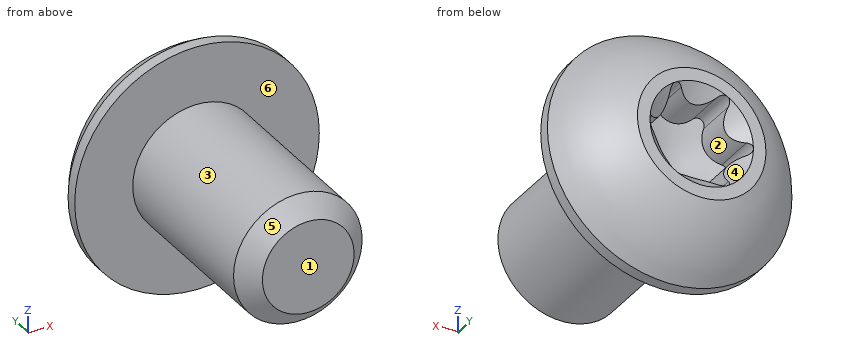
Autodesk Inventor part; units mm, degrees
ref_plane "YZ Plane" through (0, 0, 0) normal (1, 0, 0) x (0, 1, 0)
ref_plane "XZ Plane" through (0, 0, 0) normal (0, 1, 0) x (-1, 0, 0)
ref_plane "XY Plane" through (0, 0, 0) normal (0, 0, 1) x (1, 0, 0)
sketch "Sketch1" plane through (0, 0, 0) normal (0, 1, 0) x (-1, 0, 0)
  circle A0 centre (0, 0) radius 2.0828
  dimension "d4" = 4.1656
extrude "Body" add sketch "Sketch1" along normal blind 6.35
sketch "Sketch2" plane through (0, 0, 0) normal (1, 0, 0) x (0, 1, 0)
  line L0 (6.35, -2.0828) -> (6.35, 2.0828)
  line L1 (6.35, 0) -> (6.35, -3.9624)
  line L2 (6.35, -3.9624) -> (6.731, -3.9624)
  arc A0 (6.731, -3.9624) -> (8.5598, -2.0828) centre (4.5388, 0) ccw
  line L3 (8.5598, -2.0828) -> (8.5598, -1.6764)
  line L4 (8.5598, -1.6764) -> (7.0635, -1.6764)
  line L5 (7.0635, -1.6764) -> (6.4516, 0)
  line L6 (6.4516, 0) -> (6.35, 0)
  point P0 (0, 0)
  dimension "d5" = 3.9624
  dimension "d6" = 0.381
  dimension "d13" = 0.1016
  dimension "d14" = 2.0828
  dimension "d15" = 2.2098
  dimension "d16" = 0
  dimension "d17" = 1.6764
  dimension "d57" = 20.053
revolve "Head" add sketch "Sketch2" angle 360 about axis through (0, 6.4516, 0) along (0, -1, 0)
sketch "Sketch3" plane through (0, 8.5598, 0) normal (0, 1, 0) x (1, 0, 0)
  circle A0 centre (0, 0) radius 1.6764
  line L0 (0.7302, -1.2648) -> (-0.7303, -1.2648) construction
  line L1 (-0.7303, -1.2648) -> (-1.4605, 0) construction
  line L2 (-1.4605, 0) -> (-0.7303, 1.2648) construction
  line L3 (-0.7303, 1.2648) -> (0.7302, 1.2648) construction
  line L4 (0.7302, 1.2648) -> (1.4605, 0) construction
  line L5 (1.4605, 0) -> (0.7302, -1.2648) construction
  circle A1 centre (-0.7303, -1.2648) radius 0.2159
  circle A2 centre (-1.4605, 0) radius 0.2159
  circle A3 centre (-0.7303, 1.2648) radius 0.2159
  circle A4 centre (0.7302, 1.2648) radius 0.2159
  circle A5 centre (1.4605, 0) radius 0.2159
  circle A6 centre (0.7302, -1.2648) radius 0.2159
  circle A7 centre (0, -2.0701) radius 0.8712
  circle A8 centre (0, 2.0701) radius 0.8712
  circle A9 centre (1.7928, -1.0351) radius 0.8712
  circle A10 centre (-1.7928, 1.035) radius 0.8712
  circle A11 centre (1.7928, 1.035) radius 0.8712
  circle A12 centre (-1.7928, -1.0351) radius 0.8712
  circle A13 centre (0, 0) radius 1.8188
  point P0 (0, 0)
  point P1 (0, 0)
  point P2 (0.9413, 1.2192)
  point P3 (1.5265, 0.2056)
  point P4 (1.5265, -0.2056)
  point P5 (0.9413, -1.2192)
  point P6 (0.5852, -1.4248)
  point P7 (-0.5852, -1.4248)
  point P8 (-0.9413, -1.2192)
  point P9 (-1.5265, -0.2056)
  point P10 (-1.5265, 0.2056)
  point P11 (-0.9413, 1.2192)
  point P12 (-0.5852, 1.4248)
  point P13 (0.5852, 1.4248)
  dimension "d58" = 2.921
  dimension "d59" = 4.1402
  dimension "d62" = 120
extrude "Hex" add sketch "Sketch3" against normal blind 1.778 contours A5 A11 A0 | A0 A11 A13 A9 | A0 A9 A5 | A11 A0 | A0 A11 A13 | A9 A13 A0 | A0 A9 | A11 A4 A0 | A0 A8 A13 A11 | A9 A13 A7 A0 | A0 A6 A9 | A4 A8 A0 | A0 A7 A6 | A8 A0 | A7 A0 | A0 A8 A13 | A7 A13 A0 | A3 A0 A8 | A7 A0 A1 | A0 A10 A13 A8 | A7 A13 A12 A0 | A3 A10 A0 | A0 A12 A1 | A10 A0 A13 | A13 A12 A0 | A10 A0 | A0 A12 | A10 A0 A12 A13 | A10 A2 A0 | A0 A2 A12
sketch "Sketch4" plane through (0, 0, 0) normal (0, 0, 1) x (1, 0, 0)
  line L0 (-0.7364, 7.6198) -> (-1.6764, 8.5598)
  line L1 (0, 8.5598) -> (-0.7364, 7.6198)
  line L2 (0, -3.617) -> (0, 21.7018)
  line L3 (-1.5265, 8.5598) -> (-1.5265, 7.0138)
  line L4 (-1.5265, 8.5598) -> (-1.5265, 8.5598)
  line L5 (-1.5265, 8.5598) -> (-1.5265, 7.0138)
  line L6 (-1.6764, 8.5598) -> (-1.5265, 8.5598)
  line L7 (-1.6764, 8.5598) -> (0, 8.5598)
  point P0 (0, 0)
  point P1 (-1.6764, 7.0635)
  dimension "d29" = 1.6764
revolve "Head Chamfer" cut sketch "Sketch4" angle 360 about axis through (0, -10, 0) along (0, 1, 0)
sketch "Sketch5" plane through (0, 0, 0) normal (1, 0, 0) x (0, 1, 0)
  line L0 (0, -2.0828) -> (6.35, -2.0828)
  line L1 (6.35, 3.9624) -> (6.35, -3.9624)
  line L2 (6.35, -2.0828) -> (6.35, 2.0828)
  line L3 (0.0745, -2.0828) -> (-0.2261, -2.6035)
  line L4 (-0.2261, -2.6035) -> (-0.3253, -2.6035)
  line L5 (-0.3253, -2.6035) -> (-0.626, -2.0828)
  line L6 (0.0686, -2.6035) -> (-0.7252, -2.6035) construction
  line L7 (-0.626, -2.0828) -> (0.0745, -2.0828)
  line L8 (0, -2.0828) -> (6.35, -2.0828)
  point P0 (0, 0)
  dimension "d31" = 30
  dimension "d32" = 60
  dimension "a" = 0.0992
  dimension "d46" = 0.7937
  dimension "d54" = 0.0686
  dimension "d55" = 0.5207
  dimension "d56" = 0.0992
feature "Thread" [suppressed]
sketch "Sketch6" plane through (0, 0, 0) normal (0, 0, 1) x (1, 0, 0)
  line L0 (0, 0) -> (-1.4859, 0)
  line L1 (2.0828, 0) -> (-2.0828, 0)
  line L2 (-1.4859, 0) -> (-2.4948, 1.0089)
  line L3 (-2.4948, 1.0089) -> (-2.9651, -1.2188)
  line L4 (-2.9651, -1.2188) -> (-1.4859, -1.2188)
  line L5 (-2.0828, 0) -> (-2.0828, 6.35)
  line L6 (-1.4859, -1.2188) -> (-1.4859, 0)
  line L7 (0, -4.6376) -> (0, 19.2938)
  point P0 (-2.0828, 0.5969)
  dimension "d49" = 1.4859
  dimension "d50" = 135
revolve "Tapered End" cut sketch "Sketch6" angle 360 about axis through (0, -10, 0) along (0, 1, 0)
equation "\"d56\" = a"
properties part number "Screw 8-32 Steel 2.500" material "VEX Steel"
The listing builds one solid part. Answer for the finished solid, in the listing's coordinates (mm). Face numbers are marked on the shaded views. A direction names the side the tool comes from. Coordinates: 2 decimals unless noted, no trailing zeros. Write each loop counter-clockwise with the first axis right and the second up, starting at its lowest first coordinate (ties: lowest second). Pieces come first, ordered by that corner, then holes. Notation, with made-up numbers: M 19.5,89.5 L 35.5,89.5 A23 cw 35.5,98.5 Z; hole C 78,42.25 d3. An arc over 180 degrees is marked long. Use a Markdown table: item, result. Add a question column.
1. Given P1, Ø1.5, axis at x = 1, y = 4, coming from the -Z side; P2, Ø3, axis at x = 3, y = 7, coming from the +Z side; P3, Ø2, axis at x = 1.5, y = 6.5, coming from the +Z side, each flat-ended and moving along its own axis, determine where each tip first touches the part or whether it passes through.
2. Section A-A (y = 4.5) is taken. Give the vertices of the cut face in (x, z), plus the area to 3 significant figures.
3. Which of the six approach directions +Z, -Z, +X, -X, +Y, -Y give full straight-line access (tool end or side, diameter ignored) to the marked faces 1, 2 and 3?
4. For a pull along X with two mould halves and no side action, classify the marked faces 4, 5 and 6 as +X half, -X half, draft (parallel to the pull), parting line (faces both ways), or undercut.
5. Straight lines are drawn through the part: line 1 along Z through (x, y) = (0, 1.75); line 2 along X through (y, z) = (4.5, -0.5); line 3 along X through (y, z) = (0.5, 1.25). For each, find the intervals that lie inside material, in ascending order. Write a range as [from, to].
Data:
| question | item | result |
|---|---|---|
| 1 | P1 | stops at z = -2.07 |
| 1 | P2 | stops at z = 3.66 |
| 1 | P3 | stops at z = 3.93 |
| 2 | outline | C 0,0 d4.17 |
| 2 | area | 13.6 mm2 |
| 3 | face 1 | +Z, -Z, +X, -X, -Y |
| 3 | face 2 | +Y |
| 3 | face 3 | -Y |
| 4 | face 4 | undercut |
| 4 | face 5 | parting line |
| 4 | face 6 | draft |
| 5 | line 1 | z = [-2.08, 2.08] |
| 5 | line 2 | x = [-2.02, 2.02] |
| 5 | line 3 | x = [-1.54, 1.54] |
